from build123d import *

# Parameters (mm, degrees)
SKETCH_1_R      = 60
SKETCH_1_R_2    = 14.438127561
EXTRUDE_1_DEPTH = 40
CHAMFER_1_SIZE  = 2


with BuildPart() as part:
    # 草图1 → 凸台-拉伸1 (new body)
    with BuildSketch(Plane.XY.offset(70.26)):
        with Locations((-297.670899951, 626.415366791)):
            Circle(SKETCH_1_R)
        with Locations((-297.670899951, 626.415366791)):
            Circle(SKETCH_1_R_2, mode=Mode.SUBTRACT)
    extrude(amount=-EXTRUDE_1_DEPTH)

    # 草图4 → 切除-旋转1 (revolve, cut)
    with BuildSketch(Plane(origin=(0, 626.415366791, 0), x_dir=(1, 0, 0), z_dir=(0, 1, 0))):
        with BuildLine():
            Line((-244.095308656, -48.103310059), (-244.095308655, -52.416689982))
            ThreePointArc((-244.095308655, -52.416689982), (-242.284199059, -57.48597347), (-237.670899813, -60.259999987))
            Line((-237.670899813, -60.259999987), (-237.670899811, -40.260000013))
            ThreePointArc((-237.670899811, -40.260000013), (-242.284199071, -43.034026546), (-244.095308656, -48.103310059))
        make_face()
    revolve(axis=Axis((-299.491656028, 626.415366791, 70.26), (0, 0, -1)), mode=Mode.SUBTRACT)

    # 倒角1
    chamfer_1_edges = [part.edges().sort_by_distance(p)[0] for p in [
        (-357.670899951, 626.415366791, 70.26),
        (-357.670899951, 626.415366791, 30.26),
    ]]
    chamfer(chamfer_1_edges, length=CHAMFER_1_SIZE)


solid = part.part
Can you work these out from the model? Positions are in its coordinate system, mm. A direction names the side the tool comes from. Round coordinates to 2 decimals unless told otherwise and drop trailing zeros. Write each loop counter-clockwise with the first axis right and the second up, starting at its lowest first coordinate (ties: lowest second). Pieces come first, ordered by that corner, then holes. Notation, with made-up numbers: M -14,84.25 L 2,84.25 A32 cw 2,112.25 Z; hole C -31.5,26.5 d9. An arc over 180 degrees is marked long. Use CSV: the item, a comma, the result in double quotes.
(1) Imagine slicing it at A-A (z = 55.5). Write out the boundary of the cut face in (x, y).
Check values:
outline,"C -299.49,626.42 d112.03; hole C -297.67,626.42 d28.88"
(2) I need wall thicknesses on line 1 along X through (y, z) = (616.5, 65.5); line 2 along Y through (x, z) = (-279, 66.5); line 3 along Y through (x, z) = (-291, 67.5). Which ranges of each line are inside material? Lowest first, please.
Check values:
line 1,"-356.85 to -308.17, -287.18 to -238.5"
line 2,"569.39 to 683.44"
line 3,"566.79 to 613.61, 639.22 to 686.04"
(3) We'd pull the mould along Y, two halves only. Please class faces 1 (the flat face through (-286, 614, 30.26)), 2 (the cylindrical face through (-308.312, 636.173, 50.54)), 3 (the cylindrical face through (-357.613, 629.053, 37.218)): +Y half, -Y half, draft (parallel to the pull), parting line (faces both ways), or undercut.
Check values:
face 1,"draft"
face 2,"undercut"
face 3,"parting line"
(4) Imagine slicing it at B-B (z = 46). Write out the boundary of the cut face in (x, y), plus the area to 3 significant figures.
Check values:
outline,"C -299.49,626.42 d111.36; hole C -297.67,626.42 d28.88"
area,"9,080 mm^2"
(5) On a 3-axis mill with a long thin cutter (end or side, diameter ignored), from which of +Z, -Z, +X, -X, +Y, -Y can I reach the whole of each face in a straight line? I mean faces 4 (the flat face through (-286, 614, 70.26)), 5 (the cylindrical face through (-311.5, 680.494, 50.29)). Say none if no direction works.
Check values:
face 4,"+Z, +X, -X, +Y, -Y"
face 5,"none"
(6) I'm going to push flat-ended pins straight in: pin 1 (2 mm diameter, centred on x = -319, z = 55, fed in from +Y); pin 2 (5 mm diameter, centred on x = -310.5, z = 39, fed in from -Y); pin 3 (6 mm diameter, centred on y = 623, z = 35.5, fed in from -X); pin 4 (17.5 mm diameter, centred on x = -297.67, y = 626.42, fed in from +Z). Where does each tip first touch, or does it pass through?
Check values:
pin 1,"y = 679.28"
pin 2,"y = 567.31"
pin 3,"x = -357.67"
pin 4,"through"
